from build123d import *

# Parameters (mm, degrees)
SKETCH1_R       = 3.4
EXTRUDE1_DEPTH  = 16
LPATTERN2_COUNT = 6
LPATTERN2_PITCH = 1


with BuildPart() as part:
    # Sketch1 → Extrude1 (new body)
    with BuildSketch(Plane.XY):
        Polygon((8.082903769, 0), (4.041451884, 7), (-4.041451884, 7), (-8.082903769, 0), (-4.041451884, -7), (4.041451884, -7), align=None)
        Circle(SKETCH1_R, mode=Mode.SUBTRACT)
    extrude(amount=EXTRUDE1_DEPTH)

    # Sketch2 → Cut-Revolve1 (revolve, cut)
    with BuildSketch(Plane(origin=(0, 0, 0), x_dir=(1, 0, 0), z_dir=(0, 1, 0))):
        with BuildLine():
            Line((5.75, -4.5), (5.75, -12.6))
            ThreePointArc((5.75, -12.6), (5.867157288, -12.882842712), (6.15, -13))
            Line((6.15, -13), (8.082903769, -13))
            Line((8.082903769, -13), (8.082903769, 0))
            Line((8.082903769, 0), (5, 0))
            Line((5, 0), (5.25, -0.433012702))
            Line((5.25, -0.433012702), (5.25, -4))
            Line((5.25, -4), (5.75, -4.5))
        make_face()
    revolve(axis=Axis((0, 0, 0), (0, 0, 1)), mode=Mode.SUBTRACT)

    # Sketch4 → Cut-Revolve2 (revolve, cut)
    with BuildSketch(Plane(origin=(0, 0, 0), x_dir=(1, 0, 0), z_dir=(0, 1, 0))):
        Polygon((5.75, -4.5), (5.75, -5.5), (5.25, -5), align=None)
    cut_revolve2 = revolve(axis=Axis((0, 0, 0), (0, 0, 1)), mode=Mode.SUBTRACT)

    # LPattern2: Cut-Revolve2 ×6
    with Locations(*[(0, 0, i * LPATTERN2_PITCH) for i in range(1, LPATTERN2_COUNT)]):
        add(cut_revolve2, mode=Mode.SUBTRACT)


solid = part.part
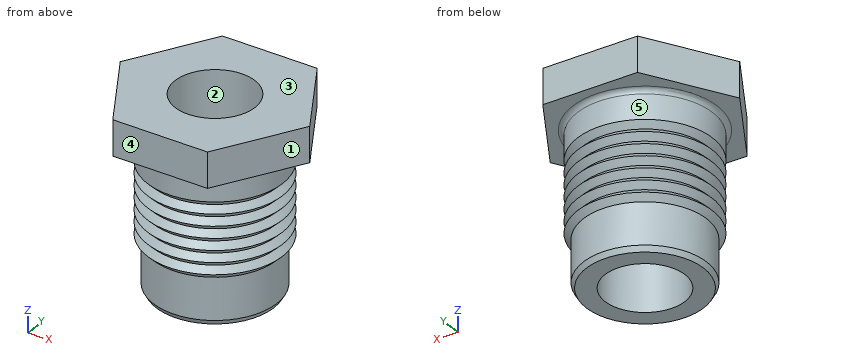
The listing builds one solid part. Answer for the finished solid, in the listing's coordinates (mm). Face numbers are marked on the shaded views. A direction names the side the tool comes from. Give positions to 0.01 mm unless a question says otherwise; leave off trailing zeros. Loops run counter-clockwise (first coordinate to the right, second up) from the corner with the lowest first, then second, coordinate; pieces in that order, holes last. Notation, with made-up numbers: (80, 63) - (111, 63) arc R10 ccw to (111, 79) - close; hole circle Ø8 at (61.5, 44.25). An arc over 180 degrees is marked (long way). Use one line per item in the form item = value.
1. Find the intervals of material crossed by line 1 along Z through (x, y) = (4.5, -4.25); line 2 along Y through (x, z) = (0, 3.75); line 3 along Y through (x, z) = (-0.75, 14.25), in increasing order. Write a range as [from, to].
Calculated:
line_1 = [13, 16]
line_2 = [-5.25, -3.4], [3.4, 5.25]
line_3 = [-7, -3.32], [3.32, 7]
2. Given pin 1 Ø1.5 at (y, z) = (-3, 11) entering from -X; pin 2 Ø1 at (x, z) = (5, 10) entering from -Y; pin 3 Ø1 at (x, z) = (3.5, 10.5) entering from -Y, each flat-ended and moving along its own axis, determine where each tip first touches the part or whether it passes through.
Calculated:
pin_1 = -5.29
pin_2 = -3.14
pin_3 = -4.91
3. The mould has two halves that part along X. Classify the marked faces 1, 2 and 3: pulls with the +X half, pulls with the -X half, needs draft (parallel to the pull), parting line crosses it, or undercut.
Calculated:
face_1 = pulls with the +X half
face_2 = undercut
face_3 = needs draft
4. Which of the six approach directions +Z, -Z, +X, -X, +Y, -Y give full straight-line access (tool end or side, diameter ignored) to the marked faces 4 and 5?
Calculated:
face_4 = +Z, -Z, +X, -X, -Y
face_5 = -Z
5. Section A-A on z = 3 is taken. Give the vertices of the cut face in (x, y).
Calculated:
outline = circle Ø10.5 at (0, 0); hole circle Ø6.8 at (0, 0)
